Autodesk Inventor part; units mm, degrees
ref_plane "YZ Plane" through (0, 0, 0) normal (1, 0, 0) x (0, 1, 0)
ref_plane "XZ Plane" through (0, 0, 0) normal (0, 1, 0) x (-1, 0, 0)
ref_plane "XY Plane" through (0, 0, 0) normal (0, 0, 1) x (1, 0, 0)
sketch "Sketch1" plane through (0, 0, 0) normal (0, 0, 1) x (1, 0, 0)
  circle A0 centre (0, 0) radius 15.95
  circle A1 centre (0, 11) radius 1.25
  circle A2 centre (-7.7782, 7.7782) radius 1.25
  circle A3 centre (-11, 0) radius 1.25
  circle A4 centre (-7.7782, -7.7782) radius 1.25
  circle A5 centre (0, -11) radius 1.25
  circle A6 centre (7.7782, -7.7782) radius 1.25
  circle A7 centre (11, 0) radius 1.25
  circle A8 centre (7.7782, 7.7782) radius 1.25
  circle A9 centre (0, 0) radius 6
  dimension "d0" = 31.9
  dimension "d1" = 2.5
  dimension "d2" = 11
  dimension "d5" = 360
  dimension "d17" = 12
extrude "Extrusion1" add sketch "Sketch1" along normal mid plane 8
properties part number "FifthAxisShaft"
Read the model definition and answer for the solid it produces. Units are mm, in the model's axes. Coordinates: 2 decimals unless noted, no trailing zeros. Write each loop counter-clockwise with the first axis right and the second up, starting at its lowest first coordinate (ties: lowest second). Pieces come first, ordered by that corner, then holes. Notation, with made-up numbers: (80, 14) -> (121, 14) arc R21 cw to (121, 32) -> close; hole circle Ø6 at (-39, 6). An arc over 180 degrees is marked (long way). Write item = value, one per line.
(1) Section B-B on y = 0 is taken. Write down the section's boundary in (x, z), plus the area to 3 significant figures.
From the geometry:
outline = (-15.95, -4) -> (-12.25, -4) -> (-12.25, 4) -> (-15.95, 4) -> close; (-9.75, -4) -> (-6, -4) -> (-6, 4) -> (-9.75, 4) -> close; (6, -4) -> (9.75, -4) -> (9.75, 4) -> (6, 4) -> close; (12.25, -4) -> (15.95, -4) -> (15.95, 4) -> (12.25, 4) -> close
area = 119 mm2
(2) Section A-A on y = -11 is taken. Write down the section's boundary in (x, z).
From the geometry:
outline = (-11.55, -4) -> (-1.25, -4) -> (-1.25, 4) -> (-11.55, 4) -> close; (1.25, -4) -> (11.55, -4) -> (11.55, 4) -> (1.25, 4) -> close
(3) Given pin 1 Ø3 at (y, z) = (-2, 0) entering from +X; pin 2 Ø2 at (x, y) = (-7.78, -7.78) entering from -Z; pin 3 Ø1.5 at (y, z) = (12, -1) entering from +X, each flat-ended and moving along its own axis, determine where each tip first touches the part or whether it passes through.
From the geometry:
pin_1 = 15.94
pin_2 = through
pin_3 = 11.31
(4) For a pull along Y with two mould halves and no side action, classify faces 1 (the face through (15.213, 4.791, 0.056)), 2 (the face through (7, 0, 4)), 3 (the face through (6.53, 7.83, 0.06)) as +Y half, -Y half, draft (parallel to the pull), parting line (faces both ways), or undercut.
From the geometry:
face_1 = parting line
face_2 = draft
face_3 = undercut
(5) Straight lines are drawn through the part: L1, parallel to Y at x = 0, z = 1.5; L2, parallel to Y at x = 0.5, z = 2.25; L3, parallel to Y at x = -12, z = 1.25. For each, find the intervals that lie inside material, in ascending order. Write a range as from..to.
From the geometry:
L1 = -15.95..-12.25, -9.75..-6, 6..9.75, 12.25..15.95
L2 = -15.94..-12.15, -9.85..-5.98, 5.98..9.85, 12.15..15.94
L3 = -10.51..-0.75, 0.75..10.51
